Part model, mm, in its own coordinate system. A direction names the side the tool comes from. Round coordinates to 2 decimals unless told otherwise and drop trailing zeros. Loops run counter-clockwise (first coordinate to the right, second up) from the corner with the lowest first, then second, coordinate; pieces in that order, holes last. Notation, with made-up numbers: M 22,49.5 L 69,49.5 A23 ccw 69,77.5 Z; hole C 65.5,62.5 d10. An arc over 180 degrees is marked long. Answer as CSV lines item,"result". Start each with the question number.
Item 1: Band-saw the part on B-B (y = 4). Give the cut face in (x, z), and give its area (3 significant figures).
Item 2: Band-saw the part on C-C (z = -1). Give the cut face in (x, y), and give its area (3 significant figures).
Item 3: Band-saw the part on D-D (x = 9.25). Give the cut face in (y, z).
Item 4: Band-saw the part on A-A (x = 13). Give the cut face in (y, z), and give its area (3 significant figures).
Item 5: Wall check: line 1 (Z direction, x = 15.5, y = 7.75); line 2 (Y direction, x = 13, z = -10.9); line 3 (X direction, y = 4, z = -11.3). Give the ranges that are in metal, low to high.
Item 6: Mould opens along X. For faces 1 (the cylindrical face through (11.5, 4.07, -11.21)), 2 (the flat face through (22, 1, -6)), 3 (the cylindrical face through (11.5, 4.07, -0.71)), 4 (the flat face through (11, 4, 0)) say: pulls with the +X half, pulls with the -X half, needs draft (parallel to the pull), parting line crosses it, or undercut.
Item 7: Which spindle directions (+Z, -Z, +X, -X, +Y, -Y) get a long thin tool onto all of the face, cutting with end or side? Do faces 5 (the flat face through (11, 5, -1.4)), 6 (the flat face through (0, 1, -6)). Say none if no direction does.
```python
from build123d import *

# Parameters (mm, degrees)
SKETCH_1_W               = 22
SKETCH_1_H               = 9.1
SKETCH_1_H_2             = 1.4
BOTTOM_DEPTH             = 1.4
SKETCH_1_3_W             = 22
SKETCH_1_3_H             = 1.4
EXTRUDE_2_DEPTH          = 8
CUT_EXTRUDE_1_DEPTH      = 27.260426501
CUT_EXTRUDE_1_DEPTH_BACK = 27.260426501
SKETCH_2_R               = 1.5


with BuildPart() as part:
    # Sketch 1 → Bottom (new body)
    with BuildSketch(Plane(origin=(0, 0, 0), x_dir=(1, 0, 0), z_dir=(0, 1, 0))):
        with Locations((11, 5.95)):
            Rectangle(SKETCH_1_W, SKETCH_1_H)
        with Locations((11, 11.2)):
            Rectangle(SKETCH_1_W, SKETCH_1_H_2)
        with Locations((11, 0.7)):
            Rectangle(SKETCH_1_W, SKETCH_1_H_2)
    extrude(amount=BOTTOM_DEPTH)

    # Sketch 1_3 → Extrude 2 (add)
    with BuildSketch(Plane(origin=(0, 0, 0), x_dir=(1, 0, 0), z_dir=(0, 1, 0))):
        with Locations((11, 11.2)):
            Rectangle(SKETCH_1_3_W, SKETCH_1_3_H)
        with Locations((11, 0.7)):
            Rectangle(SKETCH_1_3_W, SKETCH_1_3_H)
    extrude(amount=EXTRUDE_2_DEPTH)

    # Sketch 2 → Cut-Extrude 1 (cut, two sides: drawn at the far end of the back side and taken through both)
    with BuildSketch(Plane.XY.offset(-CUT_EXTRUDE_1_DEPTH_BACK)):
        with Locations((13, 4)):
            Circle(SKETCH_2_R)
    extrude(amount=CUT_EXTRUDE_1_DEPTH + CUT_EXTRUDE_1_DEPTH_BACK, mode=Mode.SUBTRACT)


solid = part.part
```
Answer block:
1,outline,"M 0,-11.9 L 11.5,-11.9 L 11.5,-10.5 L 0,-10.5 Z; M 0,-1.4 L 11.5,-1.4 L 11.5,0 L 0,0 Z; M 14.5,-11.9 L 22,-11.9 L 22,-10.5 L 14.5,-10.5 Z; M 14.5,-1.4 L 22,-1.4 L 22,0 L 14.5,0 Z"
1,area,"53.2 mm^2"
2,outline,"M 0,0 L 22,0 L 22,8 L 0,8 Z; hole C 13,4 d3"
2,area,"169 mm^2"
3,outline,"M 0,-11.9 L 8,-11.9 L 8,-10.5 L 1.4,-10.5 L 1.4,-1.4 L 8,-1.4 L 8,0 L 0,0 Z"
4,outline,"M 0,-11.9 L 2.5,-11.9 L 2.5,-10.5 L 1.4,-10.5 L 1.4,-1.4 L 2.5,-1.4 L 2.5,0 L 0,0 Z; M 5.5,-11.9 L 8,-11.9 L 8,-10.5 L 5.5,-10.5 Z; M 5.5,-1.4 L 8,-1.4 L 8,0 L 5.5,0 Z"
4,area,"26.7 mm^2"
5,line 1,"z = -11.9 to -10.5, -1.4 to 0"
5,line 2,"y = 0 to 2.5, 5.5 to 8"
5,line 3,"x = 0 to 11.5, 14.5 to 22"
6,face 1,"undercut"
6,face 2,"pulls with the +X half"
6,face 3,"undercut"
6,face 4,"needs draft"
7,face 5,"+X, -X, +Y"
7,face 6,"+Z, -Z, -X, +Y, -Y"
